```python
from build123d import *

# Parameters (mm, degrees)
SKETCH_1_R          = 1.7
EXTRUDE_1_DEPTH     = 0.8
SKETCH_1_R_2        = 1.9
EXTRUDE_1_2_DEPTH   = 0.8
EXTRUDE_5_DEPTH     = 10
CUT_EXTRUDE_3_DEPTH = 10
CUT_EXTRUDE_4_DEPTH = 10


with BuildPart() as part:
    # Sketch 1 → Extrude 1 (new body)
    with BuildSketch(Plane(origin=(0, 0, 0), x_dir=(1, 0, 0), z_dir=(0, 1, 0))):
        with BuildLine():
            Line((0, -10), (12, -10))
            Line((12, -10), (12, 0))
            Line((12, 0), (0, 0))
            ThreePointArc((0, 0), (-2.071067812, -5), (0, -10))
        make_face()
        with Locations(Location((5, -5, 0), (0, 0, 270))):
            Circle(SKETCH_1_R, mode=Mode.SUBTRACT)
    extrude(amount=EXTRUDE_1_DEPTH)



with BuildPart() as body_2:
    # Sketch 1 → Extrude 1 2 (new body)
    with BuildSketch(Plane(origin=(0, 0, 0), x_dir=(1, 0, 0), z_dir=(0, 1, 0))):
        with BuildLine():
            Line((24, -10), (24, 0))
            Line((24, 0), (36, 0))
            ThreePointArc((36, 0), (38.071067812, -5), (36, -10))
            Line((36, -10), (24, -10))
        make_face()
        with Locations(Location((31, -5, 0), (0, 0, 270))):
            Circle(SKETCH_1_R_2, mode=Mode.SUBTRACT)
    extrude(amount=EXTRUDE_1_2_DEPTH)


with BuildPart() as part_1:
    add(part.part)

    add(body_2.part)  # Extrude 5 merges body 2
    # Sketch 2 → Extrude 5 (add)
    with BuildSketch(Plane.XY.offset(10)):
        with BuildLine():
            ThreePointArc((11.007949102, 1.622594223), (10.70184983, 1.035393399), (10.082905956, 0.8))
            Line((10.082905956, 0.8), (12, 0.8))
            ThreePointArc((12, 0.8), (18, 6.8), (24, 0.8))
            Line((24, 0.8), (25.917094044, 0.8))
            ThreePointArc((25.917094044, 0.8), (25.29815017, 1.035393399), (24.992050898, 1.622594223))
            ThreePointArc((24.992050898, 1.622594223), (18, 7.84027251), (11.007949102, 1.622594223))
        make_face()
    extrude(amount=-EXTRUDE_5_DEPTH)

    # Sketch 3 → Cut-Extrude 3 (cut)
    with BuildSketch(Plane.XY.offset(10)):
        with BuildLine():
            Line((11.2, 0), (12, 0))
            Line((12, 0), (12, 0.8))
            ThreePointArc((12, 0.8), (11.765685425, 0.234314575), (11.2, 0))
        make_face()
    extrude(amount=-CUT_EXTRUDE_3_DEPTH, mode=Mode.SUBTRACT)

    # Sketch 4 → Cut-Extrude 4 (cut)
    with BuildSketch(Plane.XY.offset(10)):
        with BuildLine():
            Line((24, 0.8), (24, 0))
            Line((24, 0), (24.8, 0))
            ThreePointArc((24.8, 0), (24.234314575, 0.234314575), (24, 0.8))
        make_face()
    extrude(amount=-CUT_EXTRUDE_4_DEPTH, mode=Mode.SUBTRACT)


solid = part_1.part
```
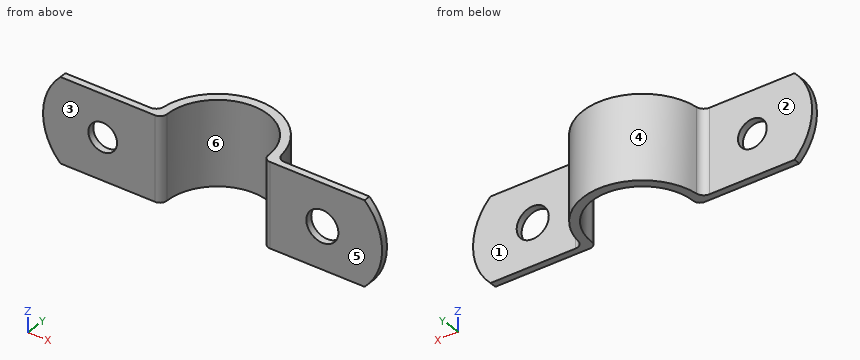
Work out the finished part from the listing and answer in its coordinate system (mm). Face numbers are marked on the shaded views. A direction names the side the tool comes from. Give positions to 0.01 mm unless a question says otherwise; leave off trailing zeros. Loops run counter-clockwise (first coordinate to the right, second up) from the corner with the lowest first, then second, coordinate; pieces in that order, holes last. Notation, with made-up numbers: (-20.5, -26) -> (-3.5, -26) arc R26 ccw to (-3.5, 11) -> close; hole circle Ø4 at (4, -27.5). An arc over 180 degrees is marked (long way). Put each result on its own line as item: value. Start each with the question number.
Item 1: The part is cut by section A-A (x = 31). Give the vertices of the cut face in (y, z).
Item 2: Find the intervals of material crossed by L1, parallel to X at y = 0.35, z = 5; L2, parallel to X at y = 0.65, z = 5; L3, parallel to Y at x = 36, z = 0.5, in increasing order. Write a range as [from, to].
Item 3: The part is cut by section B-B (z = 5). Give the vertices of the cut face in (x, y), then the cut area to 3 significant figures.
Item 4: Which of the six approach directions +Z, -Z, +X, -X, +Y, -Y give full straight-line access (tool end or side, diameter ignored) to the marked faces 1, 2 and 3?
Item 5: The part is cut by section D-D (z = 2). Give the vertices of the cut face in (x, y), then the cut area to 3 significant figures.
Item 6: Each of these flat-tipped pins is pushed along its axis until it touches: P1, Ø5, axis at x = 29, z = 5.5, coming from the +Y side; P2, Ø2, axis at y = 5, z = 5.5, coming from the +X side; P3, Ø1.5, axis at x = 25, z = 1.5, coming from the +Y side; P4, Ø1.5, axis at x = 27, y = 4.5, coming from the -Z side. Where does it stop, or does it pass through?
Item 7: The part is cut by section C-C (y = 4.5). Give the vertices of the cut face in (x, z), then the cut area to 3 significant figures.
Item 8: The mould has two halves that part along X. Classify the marked faces 4, 5 and 6: released by +X, released by -X, zero draft, split by the parting line, or undercut.
Answers below:
1. outline: (0, 0) -> (0.8, 0) -> (0.8, 3.1) -> (0, 3.1) -> close; (0, 6.9) -> (0.8, 6.9) -> (0.8, 10) -> (0, 10) -> close
2. L1: [-2.07, 3.3], [6.7, 11.86], [24.14, 29.1], [32.9, 38.07]
2. L2: [-2.07, 3.3], [6.7, 11.99], [24.01, 29.1], [32.9, 38.07]
2. L3: [0, 0.8]
3. outline: (-2.07, 0) -> (3.3, 0) -> (3.3, 0.8) -> (-2.07, 0.8) -> close; (6.7, 0) -> (11.2, 0) arc R0.8 ccw to (12, 0.8) arc R6 cw to (24, 0.8) arc R0.8 ccw to (24.8, 0) -> (29.1, 0) -> (29.1, 0.8) -> (25.92, 0.8) arc R0.93 cw to (24.99, 1.62) arc R7.04 ccw to (11.01, 1.62) arc R0.93 cw to (10.08, 0.8) -> (6.7, 0.8) -> close; (32.9, 0) -> (38.07, 0) -> (38.07, 0.8) -> (32.9, 0.8) -> close
3. area: 38.1 mm2
4. face 1: +Z, -Z, +X, +Y
4. face 2: +Z, -Z, -X, +Y
4. face 3: +Z, -Z, +X, -X, -Y
5. outline: (-1.4, 0) -> (11.2, 0) arc R0.8 ccw to (12, 0.8) arc R6 cw to (24, 0.8) arc R0.8 ccw to (24.8, 0) -> (37.4, 0) -> (37.4, 0.8) -> (25.92, 0.8) arc R0.93 cw to (24.99, 1.62) arc R7.04 ccw to (11.01, 1.62) arc R0.93 cw to (10.08, 0.8) -> (-1.4, 0.8) -> close
5. area: 42.8 mm2
6. P1: y = 0.8
6. P2: x = 24.27
6. P3: y = 4.04
6. P4: through
7. outline: (12.01, 0) -> (13.28, 0) -> (13.28, 10) -> (12.01, 10) -> close; (22.72, 0) -> (23.99, 0) -> (23.99, 10) -> (22.72, 10) -> close
7. area: 25.3 mm2
8. face 4: split by the parting line
8. face 5: zero draft
8. face 6: undercut
